from build123d import *

# Parameters (mm, degrees)
F0_W     = 660.4
F0_H     = 25.4
F1_DEPTH = 25.4
F2_W     = 50.8
F2_H     = 12.7
F3_DEPTH = 25.4
F4_W     = 558.8
F4_H     = 3.175
F5_DEPTH = 3.175


with BuildPart() as f1:
    # F0 (on Front) → F1 (new body)
    with BuildSketch(Plane.XZ):
        Rectangle(F0_W, F0_H)
    extrude(amount=F1_DEPTH)

    # F2 (on face) → F3 (cut)
    with BuildSketch(Plane.XZ.offset(25.4)):
        with Locations((-304.8, -6.35)):
            Rectangle(F2_W, F2_H)
        with Locations((304.8, -6.35)):
            Rectangle(F2_W, F2_H)
    extrude(amount=-F3_DEPTH, mode=Mode.SUBTRACT)

    # F4 (on face) → F5 (cut)
    with BuildSketch(Plane(origin=(0, 0, -12.7), x_dir=(1, 0, 0), z_dir=(0, 0, -1))):
        with Locations((0, 12.7)):
            Rectangle(F4_W, F4_H)
    extrude(amount=-F5_DEPTH, mode=Mode.SUBTRACT)


solid = f1.part
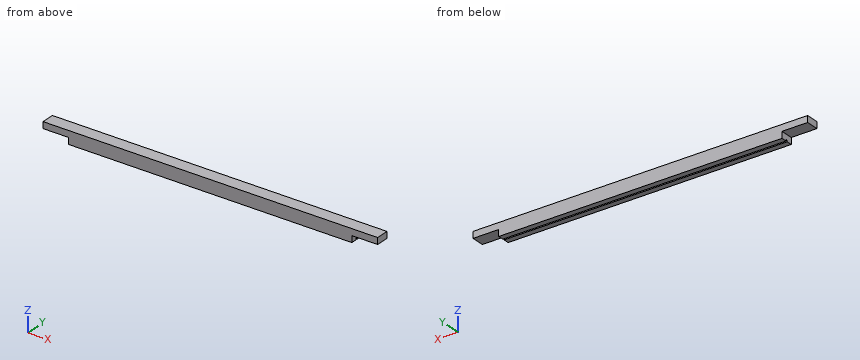
Geometry: final body of the model. Coordinates: model frame, mm. Coordinates: 2 decimals unless noted, no trailing zeros. Write each loop counter-clockwise with the first axis right and the second up, starting at its lowest first coordinate (ties: lowest second). Pieces come first, ordered by that corner, then holes. Notation, with made-up numbers: (49.5, 12) - (53.5, 12) arc R13 ccw to (53.5, 35) - close; hole circle Ø3 at (-38.75, 14.25). An arc over 180 degrees is marked (long way). Return JSON: item names as keys, results as strings.
Item 1: Section query B-B (x = -289). Output: boundary loops of the cut face in (y, z).
Completed:
{"outline": "(-25.4, 0) - (0, 0) - (0, 12.7) - (-25.4, 12.7) - close"}
Item 2: Line query: L1, parallel to Y at x = 147, z = -11.25; L2, parallel to X at y = -6.5, z = -10.25; L3, parallel to Z at x = 249.5, y = -14 (3 decimals). Output: solid intervals per line, ascending.
Completed:
{"L1": "y = -25.4 to -14.29, -11.11 to 0", "L2": "x = -279.4 to 279.4", "L3": "z = -9.525 to 12.7"}
Item 3: Pin query (flat end, axial travel): pin 1 Ø4 at (y, z) = (-9.5, -4) entering from -X; pin 2 Ø7.5 at (x, y) = (307.5, -15.5) entering from -Z; pin 3 Ø1.6 at (x, y) = (42.5, -12) entering from -Z (3 decimals). Return the tip coordinate at first contact, or that it passes through.
Completed:
{"pin 1": "stops at x = -279.4", "pin 2": "stops at z = 0", "pin 3": "stops at z = -9.525"}
Item 4: Section query A-A (x = 173). Output: boundary loops of the cut face in (y, z) (1 decimal).
Completed:
{"outline": "(-25.4, -12.7) - (-14.3, -12.7) - (-14.3, -9.5) - (-11.1, -9.5) - (-11.1, -12.7) - (0, -12.7) - (0, 12.7) - (-25.4, 12.7) - close"}
